The drawing under review shows one solid part. Ordinate dimensions are in mm from its lowest x, y, z. Give positions to 0.01 mm unless a question says otherwise; leave off trailing zeros. Write each loop counter-clockwise with the first axis right and the second up, starting at its lowest first coordinate (ties: lowest second). Pieces come first, ordered by that corner, then holes. Notation, with made-up numbers: M -35.5,57.5 L -16.5,57.5 A18 ccw -16.5,85.5 Z; hole C 39.25,-15.5 d2. An arc over 180 degrees is marked long. Write item = value, one per line. Start each with the question number.
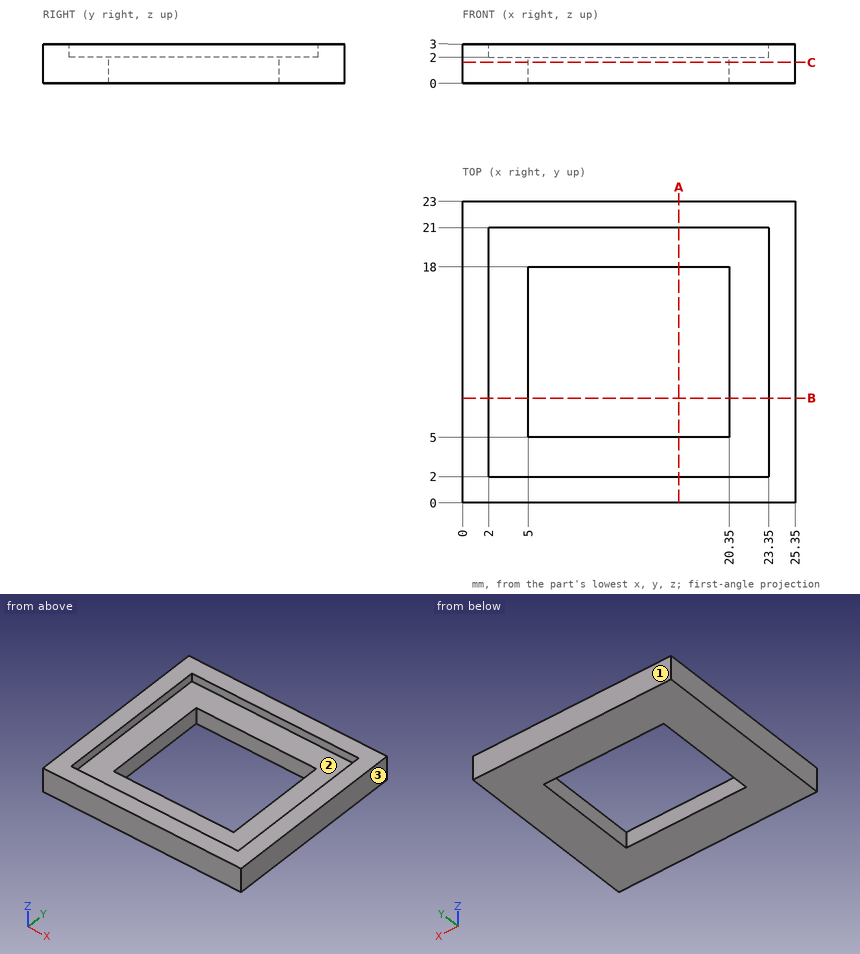
Item 1: The part is to be moulded in two halves that separate along X. For the marked faces 1, 2 and 3, say which applies: released by +X, released by -X, zero draft, split by the parting line, or undercut.
Item 2: We need section B-B, the plane y = 8. Write out the cut boundary in (x, z).
Item 3: Clearance check with a flat-ended pin moving along its axis: P1, Ø4, axis at x = 20, y = 12.5, coming from the +Z side. State where the tip first meets the part, or that it passes through.
Item 4: To check wall thickness, follow probe 1 along X at (y, z) = (8, 1.9); probe 2 along X at (y, z) = (11, 2.1); probe 3 along Y at (x, z) = (19, 2.8). State the ranges of each line that lie inside material, in increasing order. Write a range as [from, to].
Item 5: We need section A-A, the plane x = 16.5. Write out the cut boundary in (y, z).
Item 6: We need section C-C, the plane z = 1.6. Write out the cut boundary in (x, y).
Worked out:
q1.face_1 = zero draft
q1.face_2 = undercut
q1.face_3 = released by +X
q2.outline = M 0,0 L 5,0 L 5,2 L 2,2 L 2,3 L 0,3 Z; M 20.35,0 L 25.35,0 L 25.35,3 L 23.35,3 L 23.35,2 L 20.35,2 Z
q3.P1 = 2
q4.probe_1 = [0, 5], [20.35, 25.35]
q4.probe_2 = [0, 2], [23.35, 25.35]
q4.probe_3 = [0, 2], [21, 23]
q5.outline = M 0,0 L 5,0 L 5,2 L 2,2 L 2,3 L 0,3 Z; M 18,0 L 23,0 L 23,3 L 21,3 L 21,2 L 18,2 Z
q6.outline = M 0,0 L 25.35,0 L 25.35,23 L 0,23 Z; hole M 5,5 L 20.35,5 L 20.35,18 L 5,18 Z
